Here's how the part is built. I have some questions about the finished solid (model axes, mm). Face numbers are marked on the shaded views. Coordinates: 2 decimals unless noted, no trailing zeros. Write each loop counter-clockwise with the first axis right and the second up, starting at its lowest first coordinate (ties: lowest second). Pieces come first, ordered by that corner, then holes.
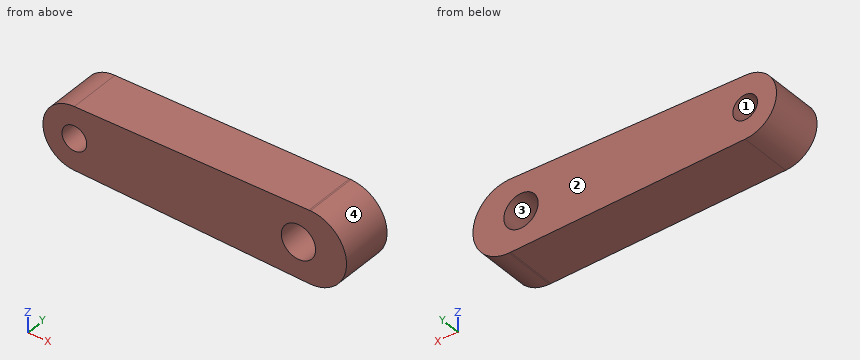
```python
from build123d import *

# Parameters (mm, degrees)
SKETCH1_R           = 6.5
SKETCH1_R_2         = 9
BOSS_EXTRUDE1_DEPTH = 27.5


with BuildPart() as part:
    # Sketch1 → Boss-Extrude1 (new body)
    with BuildSketch(Plane(origin=(0, 0, 0), x_dir=(1, 0, 0), z_dir=(0, 1, 0))):
        with BuildLine():
            ThreePointArc((124, -19), (143, 0), (124, 19))
            Line((124, 19), (123.234182256, 18.984560126))
            Line((123.234182256, 18.984560126), (0, 16.5))
            ThreePointArc((0, 16.5), (-16.5, 0), (0, -16.5))
            Line((0, -16.5), (123.234182256, -18.984560126))
            Line((123.234182256, -18.984560126), (124, -19))
        make_face()
        with Locations(Location((0, 0, 0), (0, 0, 270))):
            Circle(SKETCH1_R, mode=Mode.SUBTRACT)
        with Locations(Location((117.75, 0, 0), (0, 0, 270))):
            Circle(SKETCH1_R_2, mode=Mode.SUBTRACT)
    extrude(amount=BOSS_EXTRUDE1_DEPTH)


solid = part.part
```
1) Will these pins go through, and if not, where does the flat tip stop? pin 1 (12 mm diameter, centred on x = 75, y = 23, fed in from -Z); pin 2 (5 mm diameter, centred on y = 13, z = -11, fed in from -X); pin 3 (12 mm diameter, centred on y = 17, z = 1.5, fed in from +X); pin 4 (10 mm diameter, centred on x = 121.5, z = 0.5, fed in from +Y).
Values follow:
pin 1: stops at z = -18.13
pin 2: stops at x = -14.14
pin 3: stops at x = 143
pin 4: passes through
2) Imagine slicing it at D-D on x = 38. Please give me the cut outline in (y, z).
Values follow:
outline: (0, -17.27) - (27.5, -17.27) - (27.5, 17.27) - (0, 17.27) - close
3) Imagine slicing it at C-C on x = 117.75. Please give me the cut outline in (y, z), then the cut area to 3 significant figures.
Values follow:
outline: (0, -18.87) - (27.5, -18.87) - (27.5, -9) - (0, -9) - close; (0, 9) - (27.5, 9) - (27.5, 18.87) - (0, 18.87) - close
area: 543 mm2
4) We'd pull the mould along X, two halves only. Please class the marked faces 1, 2, 3 and 4: pulls with the +X half, pulls with the -X half, needs draft (parallel to the pull), parting line crosses it, or undercut.
Values follow:
face 1: undercut
face 2: needs draft
face 3: undercut
face 4: pulls with the +X half
5) Imagine slicing it at A-A on z = 0. Please give me the cut outline in (x, y), then the cut area to 3 significant figures.
Values follow:
outline: (-16.5, 0) - (-6.5, 0) - (-6.5, 27.5) - (-16.5, 27.5) - close; (6.5, 0) - (108.75, 0) - (108.75, 27.5) - (6.5, 27.5) - close; (126.75, 0) - (143, 0) - (143, 27.5) - (126.75, 27.5) - close
area: 3,530 mm2
6) I need wall thicknesses on probe 1 along X at (y, z) = (6.5, 0); probe 2 along X at (y, z) = (17, -6); probe 3 along Z at (x, y) = (24.5, 3). Which ranges of each line are inside material? Lowest first, please.
Values follow:
probe 1: x = -16.5 to -6.5, 6.5 to 108.75, 126.75 to 143
probe 2: x = -15.37 to -2.5, 2.5 to 111.04, 124.46 to 142.03
probe 3: z = -16.99 to 16.99
7) Imagine slicing it at B-B on y = 21.5. Please give me the cut outline in (x, z), then the cut area to 3 significant figures.
Values follow:
outline: (0, -16.5) - (124, -19) arc R19 ccw to (124, 19) - (0, 16.5) arc R16.5 ccw to start; hole circle Ø13 at (0, 0); hole circle Ø18 at (117.75, 0)
area: 5,010 mm2
